from build123d import *

# Parameters (mm, degrees)
SKETCH_1_R          = 30
EXTRUDE_1_DEPTH     = 30
SKETCH_2_R          = 29
CUT_EXTRUDE_1_DEPTH = 26
CUT_EXTRUDE_3_DEPTH = 74


with BuildPart() as part:
    # 草圖1 → 填料-伸長1 (new body)
    with BuildSketch(Plane(origin=(0, 0, 0), x_dir=(1, 0, 0), z_dir=(0, 1, 0))):
        Circle(SKETCH_1_R)
    extrude(amount=EXTRUDE_1_DEPTH)

    # 草圖2 → 除料-伸長1 (cut)
    with BuildSketch(Plane(origin=(0, 0, 0), x_dir=(1, 0, 0), z_dir=(0, 1, 0))):
        Circle(SKETCH_2_R)
    extrude(amount=CUT_EXTRUDE_1_DEPTH, mode=Mode.SUBTRACT)

    # 草圖4 → 除料-伸長3 (cut)
    with BuildSketch(Plane(origin=(0, 0, 0), x_dir=(1, 0, 0), z_dir=(0, 1, 0))):
        with BuildLine():
            Line((-20.622074934, 18.510350175), (-21.441043067, 17.691382042))
            Line((-21.441043067, 17.691382042), (-20.175275746, 16.455577197))
            Line((-20.175275746, 16.455577197), (-19.55132785, 17.175583262))
            ThreePointArc((-19.55132785, 17.175583262), (-10.748837833, 23.729884815), (-0.025402307, 26.064543216))
            ThreePointArc((-0.025402307, 26.064543216), (10.698033219, 23.729884815), (19.500523236, 17.175583262))
            Line((19.500523236, 17.175583262), (20.124471132, 16.455577197))
            Line((20.124471132, 16.455577197), (21.390238453, 17.691382042))
            Line((21.390238453, 17.691382042), (20.57127032, 18.510350175))
            ThreePointArc((20.57127032, 18.510350175), (11.290375881, 25.406586919), (-0.025402307, 27.782770163))
            ThreePointArc((-0.025402307, 27.782770163), (-11.341180495, 25.406586919), (-20.622074934, 18.510350175))
        make_face()
    extrude(amount=CUT_EXTRUDE_3_DEPTH, mode=Mode.SUBTRACT)


solid = part.part
Geometry: final body of the model. Coordinates: model frame, mm. A direction names the side the tool comes from. Give positions to 0.01 mm unless a question says otherwise; leave off trailing zeros. Order: outer loops, then holes, each group sorted by start corner. A loop starts at its lowest first (then second) coordinate and runs counter-clockwise, first axis right, second up. Notation, with made-up numbers: (18, 55) -> (51, 55) arc R17 cw to (51, 81) -> close; hole circle Ø10 at (61.5, -26.75). An arc over 180 degrees is marked (long way). Put each result on its own line as item: value.
Q1. Section D-D, the plane z = 25. Return loops of the section in (x, y), then the cut area to 3 significant figures.
Here are the results:
outline: (-16.58, 0) -> (-14.7, 0) -> (-14.7, 26) -> (14.7, 26) -> (14.7, 0) -> (16.58, 0) -> (16.58, 30) -> (-16.58, 30) -> close
area: 231 mm^2
Q2. Pin query (flat end, axial travel): pin 1 (4 mm diameter, centred on x = 4, y = 26, fed in from +Z); pin 2 (5 mm diameter, centred on y = 8.5, z = 7, fed in from -X); pin 3 (10 mm diameter, centred on x = 9, y = 23.5, fed in from +Z). Return the tip coordinate at first contact, or that it passes through.
Here are the results:
pin 1: stops at z = 29.93
pin 2: stops at x = -29.66
pin 3: stops at z = 29.73
Q3. Draft query along X for faces 1 (the face through (0, 30, 0)), 2 (the face through (0, 26, 0)), 3 (the face through (-29.97, 14.79, -1.32)). Return one class per face: released by +X, released by -X, zero draft, split by the parting line, or undercut.
Here are the results:
face 1: zero draft
face 2: undercut
face 3: split by the parting line
Q4. Section A-A, the plane x = -7. Return loops of the section in (y, z), then the cut area to 3 significant figures.
Here are the results:
outline: (0, -29.17) -> (30, -29.17) -> (30, -26.93) -> (26, -26.93) -> (26, -28.14) -> (0, -28.14) -> close; (0, 28.14) -> (26, 28.14) -> (26, -25.1) -> (30, -25.1) -> (30, 29.17) -> (0, 29.17) -> close
area: 280 mm^2
Q5. Reachability of faces 4 (the face through (13.38, 12.82, 25.73)), 5 (the face through (11.44, 27.97, -25.34)), 6 (the face through (-16, 0, -25)) from +Z, -Z, +X, -X, +Y, -Y: full face, straight path, thin tool, end or side. Return the list, or none.
Here are the results:
face 4: -Y
face 5: +Y, -Y
face 6: +Z, -Z, +X, -X, -Y
Q6. Material intervals for L1, parallel to Z at x = 0, y = 8.5; L2, parallel to Y at x = 17.5, z = -10, sorted ascending.
Here are the results:
L1: z = -30 to -29, 29 to 30
L2: y = 26 to 30
Q7. Section C-C, the plane y = 3.5. Return loops of the section in (x, z).
Here are the results:
outline: circle Ø60 at (0, 0); hole circle Ø58 at (0, 0)
Q8. Section B-B, the plane z = 0. Return loops of the section in (x, y), then the cut area to 3 significant figures.
Here are the results:
outline: (-30, 0) -> (-29, 0) -> (-29, 26) -> (29, 26) -> (29, 0) -> (30, 0) -> (30, 30) -> (-30, 30) -> close
area: 292 mm^2
